from build123d import *

# Parameters (mm, degrees)
SKETCH_1_W          = 18
SKETCH_1_H          = 18
EXTRUDE_1_DEPTH     = 35
CUT_EXTRUDE_2_DEPTH = 35


with BuildPart() as part:
    # 草图1 → 拉伸1 (new body)
    with BuildSketch(Plane.XY):
        Rectangle(SKETCH_1_W, SKETCH_1_H)
    extrude(amount=EXTRUDE_1_DEPTH)

    # 草图2 → 拉伸2 (cut)
    with BuildSketch(Plane(origin=(0, 9, 0), x_dir=(1, 0, 0), z_dir=(0, 1, 0))):
        with BuildLine():
            Line((3.85, -32), (3.85, -28.3))
            ThreePointArc((3.85, -28.3), (5.5, -26.65), (7.15, -28.3))
            Line((7.15, -28.3), (7.15, -32))
            ThreePointArc((7.15, -32), (5.5, -33.65), (3.85, -32))
        make_face()
        with BuildLine():
            Line((-7.15, -32), (-7.15, -28.3))
            ThreePointArc((-7.15, -28.3), (-5.5, -26.65), (-3.85, -28.3))
            Line((-3.85, -28.3), (-3.85, -32))
            ThreePointArc((-3.85, -32), (-5.5, -33.65), (-7.15, -32))
        make_face()
    extrude(amount=-CUT_EXTRUDE_2_DEPTH, mode=Mode.SUBTRACT)


solid = part.part
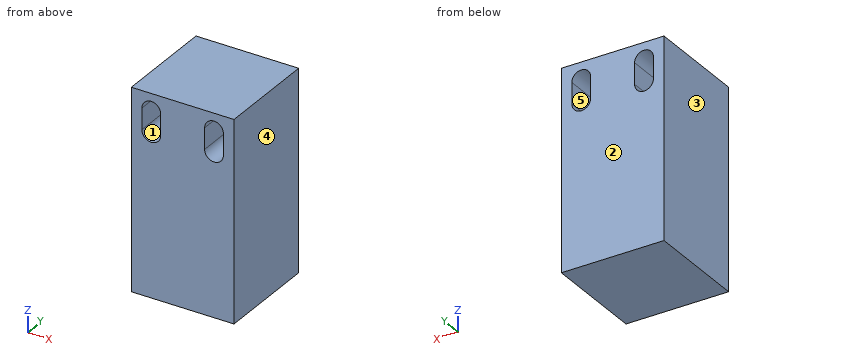
Can you work these out from the model? Positions are in its coordinate system, mm. Face numbers are marked on the shaded views. A direction names the side the tool comes from. Coordinates: 2 decimals unless noted, no trailing zeros. Loops run counter-clockwise (first coordinate to the right, second up) from the corner with the lowest first, then second, coordinate; pieces in that order, holes last. Notation, with made-up numbers: M 21.5,20.25 L 49.5,20.25 A21 ccw 49.5,28.25 Z; hole C -6.5,14.25 d5. An arc over 180 degrees is marked long. Return JSON: item names as keys, results as strings. Group by question number.
Item 1: Imagine slicing it at C-C (x = 5). Please give me the cut outline in (y, z).
Item 2: If I drill on L1, parallel to X at y = -3.75, z = 30.5; L2, parallel to Z at x = -6, y = -0.75, over which ranges is the centre line in solid material (lowest first)? Write a range as from..to.
Item 3: Imagine slicing it at B-B (y = -4.5). Please give me the cut outline in (x, z), and give its area (3 significant figures).
Item 4: Thinking about a two-plate mould opening in X: for the marked faces 3, 4 and 5, which applies, released by +X, released by -X, zero draft, split by the parting line, or undercut?
Item 5: On a 3-axis mill with a long thin cutter (end or side, diameter ignored), from which of +Z, -Z, +X, -X, +Y, -Y can I reach the whole of each face in a straight line? I mean the marked faces 1 and 2. Say none if no direction works.
Item 6: Imagine slicing it at A-A (x = -5.5). Please give me the cut outline in (y, z).
Verdict:
{
 "1": {"outline": "M -9,0 L 9,0 L 9,26.73 L -9,26.73 Z; M -9,33.57 L 9,33.57 L 9,35 L -9,35 Z"},
 "2": {"L1": "x = -9..-7.15, -3.85..3.85, 7.15..9", "L2": "z = 0..26.73, 33.57..35"},
 "3": {"outline": "M -9,0 L 9,0 L 9,35 L -9,35 Z; hole M -7.15,28.3 A1.65 ccw -3.85,28.3 L -3.85,32 A1.65 ccw -7.15,32 Z; hole M 3.85,28.3 A1.65 ccw 7.15,28.3 L 7.15,32 A1.65 ccw 3.85,32 Z", "area": "588 mm^2"},
 "4": {"face 3": "released by -X", "face 4": "released by +X", "face 5": "undercut"},
 "5": {"face 1": "+Y, -Y", "face 2": "+Z, -Z, +X, -X, +Y"},
 "6": {"outline": "M -9,0 L 9,0 L 9,26.65 L -9,26.65 Z; M -9,33.65 L 9,33.65 L 9,35 L -9,35 Z"}
}
